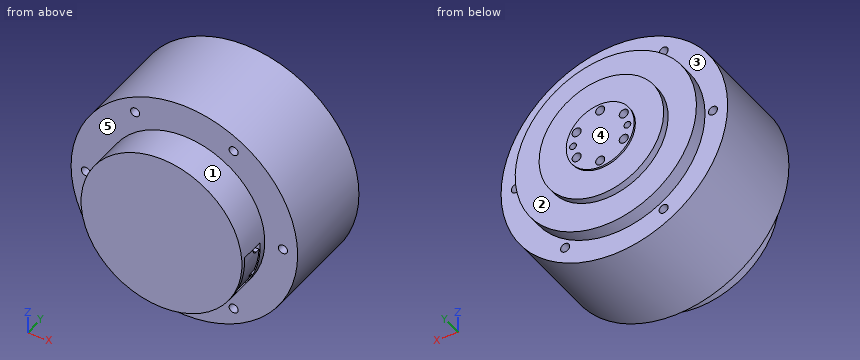
```python
from build123d import *

# Parameters (mm, degrees)
SKETCH2_R                = 35.5
BOSS_EXTRUDE1_DEPTH      = 16
SKETCH3_R                = 50
BOSS_EXTRUDE2_DEPTH      = 42.86
SKETCH4_R                = 40
BOSS_EXTRUDE3_DEPTH      = 6
SKETCH5_R                = 27.5
BOSS_EXTRUDE4_DEPTH      = 3.1
SKETCH6_R                = 15
BOSS_EXTRUDE5_DEPTH      = 0.82
SKETCH7_R                = 1.5
CUT_EXTRUDE1_DEPTH       = 3
SKETCH8_R                = 2
CUT_EXTRUDE2_DEPTH       = 8
SKETCH9_R                = 2
CUT_EXTRUDE3_DEPTH       = 8.5
CUT_EXTRUDE4_START       = -4.5
SKETCH10_R               = 2
CUT_EXTRUDE4_DEPTH       = 4.5
SKETCH12_W               = 22
SKETCH12_H               = 11
CUT_EXTRUDE6_DEPTH       = 54.5
BOSS_EXTRUDE6_REACH      = 100.644
BOSS_EXTRUDE6_END_RADIUS = 35


with BuildPart() as part:
    # Sketch2 → Boss-Extrude1 (new body)
    with BuildSketch(Plane(origin=(0, 0, 0), x_dir=(1, 0, 0), z_dir=(0, 1, 0))):
        with Locations(Location((0, 0, 0), (0, 0, 270))):
            Circle(SKETCH2_R)
    extrude(amount=BOSS_EXTRUDE1_DEPTH)

    # Sketch3 → Boss-Extrude2 (add)
    with BuildSketch(Plane(origin=(0, 16, 0), x_dir=(1, 0, 0), z_dir=(0, 1, 0))):
        with Locations(Location((0, 0, 0), (0, 0, 270))):
            Circle(SKETCH3_R)
    extrude(amount=BOSS_EXTRUDE2_DEPTH)

    # Sketch4 → Boss-Extrude3 (add)
    with BuildSketch(Plane(origin=(0, 58.86, 0), x_dir=(1, 0, 0), z_dir=(0, 1, 0))):
        with Locations(Location((0, 0, 0), (0, 0, 270))):
            Circle(SKETCH4_R)
    extrude(amount=BOSS_EXTRUDE3_DEPTH)

    # Sketch5 → Boss-Extrude4 (add)
    with BuildSketch(Plane(origin=(0, 64.86, 0), x_dir=(1, 0, 0), z_dir=(0, 1, 0))):
        with Locations(Location((0, 0, 0), (0, 0, 90))):
            Circle(SKETCH5_R)
    extrude(amount=BOSS_EXTRUDE4_DEPTH)

    # Sketch6 → Boss-Extrude5 (add)
    with BuildSketch(Plane(origin=(0, 67.96, 0), x_dir=(1, 0, 0), z_dir=(0, 1, 0))):
        with Locations(Location((0, 0, 0), (0, 0, 270))):
            Circle(SKETCH6_R)
    extrude(amount=BOSS_EXTRUDE5_DEPTH)

    # Sketch7 → Cut-Extrude1 (cut)
    with BuildSketch(Plane(origin=(0, 68.78, 0), x_dir=(1, 0, 0), z_dir=(0, 1, 0))):
        with Locations(Location((12, 0, 0), (0, 0, 270))):
            Circle(SKETCH7_R)
        with Locations(Location((-12, 0, 0), (0, 0, 270))):
            Circle(SKETCH7_R)
    extrude(amount=-CUT_EXTRUDE1_DEPTH, mode=Mode.SUBTRACT)

    # Sketch8 → Cut-Extrude2 (cut)
    with BuildSketch(Plane(origin=(0, 68.78, 0), x_dir=(1, 0, 0), z_dir=(0, 1, 0))):
        with Locations(Location((10.392304845, -6, 0), (0, 0, 270))):
            Circle(SKETCH8_R)
        with Locations(Location((0, -12, 0), (0, 0, 270))):
            Circle(SKETCH8_R)
        with Locations(Location((-10.392304845, -6, 0), (0, 0, 270))):
            Circle(SKETCH8_R)
        with Locations(Location((-10.392304845, 6, 0), (0, 0, 270))):
            Circle(SKETCH8_R)
        with Locations(Location((0, 12, 0), (0, 0, 270))):
            Circle(SKETCH8_R)
        with Locations(Location((10.392304845, 6, 0), (0, 0, 270))):
            Circle(SKETCH8_R)
    extrude(amount=-CUT_EXTRUDE2_DEPTH, mode=Mode.SUBTRACT)

    # Sketch9 → Cut-Extrude3 (cut)
    with BuildSketch(Plane(origin=(0, 58.86, 0), x_dir=(1, 0, 0), z_dir=(0, 1, 0))):
        with Locations(Location((43.5, 0, 0), (0, 0, 270))):
            Circle(SKETCH9_R)
        with Locations(Location((21.75, -37.672105065, 0), (0, 0, 270))):
            Circle(SKETCH9_R)
        with Locations(Location((-21.75, -37.672105065, 0), (0, 0, 270))):
            Circle(SKETCH9_R)
        with Locations(Location((-43.5, 0, 0), (0, 0, 270))):
            Circle(SKETCH9_R)
        with Locations(Location((-21.75, 37.672105065, 0), (0, 0, 270))):
            Circle(SKETCH9_R)
        with Locations(Location((21.75, 37.672105065, 0), (0, 0, 270))):
            Circle(SKETCH9_R)
    extrude(amount=-CUT_EXTRUDE3_DEPTH, mode=Mode.SUBTRACT)

    # Sketch10 → Cut-Extrude4 (cut)
    with BuildSketch(Plane.XZ.offset(-16).offset(CUT_EXTRUDE4_START)):
        with Locations(Location((-43.5, 0, 0), (0, 0, 90))):
            Circle(SKETCH10_R)
        with Locations(Location((-21.75, 37.672105065, 0), (0, 0, 90))):
            Circle(SKETCH10_R)
        with Locations(Location((21.75, 37.672105065, 0), (0, 0, 90))):
            Circle(SKETCH10_R)
        with Locations(Location((43.5, 0, 0), (0, 0, 90))):
            Circle(SKETCH10_R)
        with Locations(Location((21.75, -37.672105065, 0), (0, 0, 90))):
            Circle(SKETCH10_R)
        with Locations(Location((-21.75, -37.672105065, 0), (0, 0, 90))):
            Circle(SKETCH10_R)
    extrude(amount=CUT_EXTRUDE4_DEPTH, mode=Mode.SUBTRACT)

    # Sketch12 → Cut-Extrude6 (cut)
    with BuildSketch(Plane(origin=(0, 0, 0), x_dir=(0, 0, -1), z_dir=(1, 0, 0))):
        with Locations((9, 7.3)):
            Rectangle(SKETCH12_W, SKETCH12_H)
    extrude(amount=CUT_EXTRUDE6_DEPTH, mode=Mode.SUBTRACT)

    # Boss-Extrude6: up to this cylinder (the profile starts inside it)
    boss_extrude6_end = Plane(origin=(0, 6.970651, 0), z_dir=(0, -1, 0)) * Cylinder(BOSS_EXTRUDE6_END_RADIUS, 272.288, mode=Mode.PRIVATE)
    # Sketch13 → Boss-Extrude6 (add, up to the surface)
    with BuildSketch(Plane(origin=(0, 0, 0), x_dir=(0, 0, -1), z_dir=(1, 0, 0)), mode=Mode.PRIVATE) as boss_extrude6_sk1:
        with BuildLine():
            Line((1.425115379, 10.619463885), (1.425115379, 12.8))
            Line((1.425115379, 12.8), (12.035760987, 12.8))
            Line((12.035760987, 12.8), (12.035760987, 11.49))
            ThreePointArc((12.035760987, 11.49), (13.345760987, 10.18), (14.655760987, 11.49))
            Line((14.655760987, 11.49), (14.655760987, 12.8))
            Line((14.655760987, 12.8), (20, 12.8))
            Line((20, 12.8), (20, 1.8))
            Line((20, 1.8), (-2, 1.8))
            Line((-2, 1.8), (-2, 9.216236834))
            ThreePointArc((-2, 9.216236834), (0.183326841, 8.768757161), (1.425115379, 10.619463885))
        make_face()
    boss_extrude6_tool1 = extrude(boss_extrude6_sk1.sketch, amount=BOSS_EXTRUDE6_REACH, mode=Mode.PRIVATE) & boss_extrude6_end
    add(boss_extrude6_tool1.solids().sort_by_distance((0, 6.970651, -9.434063))[0])


solid = part.part
```
Verification items for the finished model (mm, model axes). Face numbers are marked on the shaded views. A direction names the side the tool comes from. Coordinates: 2 decimals unless noted, no trailing zeros. Order: outer loops, then holes, each group sorted by start corner. A loop starts at its lowest first (then second) coordinate and runs counter-clockwise, first axis right, second up. Notation, with made-up numbers: (20, -16) -> (32, -16) arc R7 cw to (32, -11) -> close; hole circle Ø8 at (50, -12.75). An arc over 180 degrees is marked (long way). Answer as CSV lines item,"result". Start each with the question number.
1) Cross-section at A-A, the plane y = 63. Record the boundary of the cut face in (x, z).
2) Cross-section at B-B, the plane x = -30. Record the boundary of the cut face in (y, z).
3) Gauge pin test, flat ends, axial feed: pin 1 Ø3 at (x, z) = (-10.39, 6) entering from -Y; pin 2 Ø4.5 at (x, z) = (21.75, -37.67) entering from -Y; pin 3 Ø2.5 at (x, y) = (10.5, 11) entering from +Z; pin 4 Ø1 at (y, z) = (15, -4.5) entering from -X. Record the tip position at first contact, or that the pin passes through.
4) Cross-section at D-D, the plane y = 22. Record the boundary of the cut face in (x, z), then the cut area to 3 significant figures.
5) Cross-section at C-C, the plane z = 12. Record the boundary of the cut face in (x, y), then the cut area to 3 significant figures.
6) Release check for a two-part mould opening along Z. For the marked faces 1 and 2 record: released by +Z, released by -Z, zero draft, split by the parting line, or undercut.
7) Set-up check for the marked faces 3, 4 and 5: record each of +Z, -Z, +X, -X, +Y, -Y from which the full face is reachable in a straight line by a thin tool's end or side.
8) Material ranges on L1, parallel to X at y = 67.85, z = 0; L2, parallel to Z at x = -21, y = 17; L3, parallel to Y at x = -9, z = -19.5, recorded low to high. Write a range as [from, to].
Conclusion:
1,outline,"circle Ø80 at (0, 0); hole circle Ø4 at (-10.39, -6); hole circle Ø4 at (-10.39, 6); hole circle Ø4 at (0, -12); hole circle Ø4 at (0, 12); hole circle Ø4 at (10.39, -6); hole circle Ø4 at (10.39, 6)"
2,outline,"(0, -18.98) -> (16, -18.98) -> (16, -40) -> (58.86, -40) -> (58.86, -26.46) -> (64.86, -26.46) -> (64.86, 26.46) -> (58.86, 26.46) -> (58.86, 40) -> (16, 40) -> (16, 18.98) -> (0, 18.98) -> close"
3,pin 1,"stops at y = 0"
3,pin 2,"stops at y = 16"
3,pin 3,"stops at z = 34.27"
3,pin 4,"stops at x = -35.27"
4,outline,"circle Ø100 at (0, 0)"
4,area,"7,850 mm²"
5,outline,"(-48.54, 16) -> (-33.41, 16) -> (-33.41, 0) -> (33.41, 0) -> (33.41, 16) -> (48.54, 16) -> (48.54, 58.86) -> (38.16, 58.86) -> (38.16, 64.86) -> (24.74, 64.86) -> (24.74, 67.96) -> (9, 67.96) -> (9, 68.78) -> (2, 68.78) -> (2, 60.78) -> (-2, 60.78) -> (-2, 68.78) -> (-9, 68.78) -> (-9, 67.96) -> (-24.74, 67.96) -> (-24.74, 64.86) -> (-38.16, 64.86) -> (-38.16, 58.86) -> (-48.54, 58.86) -> close"
5,area,"5,820 mm²"
6,face 1,"split by the parting line"
6,face 2,"zero draft"
7,face 3,"+Y"
7,face 4,"+Z, -Z, +X, -X, +Y"
7,face 5,"-Y"
8,L1,"x = [-27.5, -13.5], [-10.5, 10.5], [13.5, 27.5]"
8,L2,"z = [-45.38, -39.53], [-35.82, 35.82], [39.53, 45.38]"
8,L3,"y = [0, 67.96]"
